from build123d import *

# Parameters (mm, degrees)
SKETCH_1_R          = 1.621125
EXTRUDE_403_DEPTH   = 3.2
SKETCH_2_OUTSIDE_W  = 36.28
SKETCH_2_OUTSIDE_H  = 37.362
SKETCH_2_OUTSIDE_R  = 3.5
CUT_EXTRUDE_1_DEPTH = 7.23083729
CUT_EXTRUDE_1_DRAFT = -60
SKETCH_3_OUTSIDE_W  = 36.28
SKETCH_3_OUTSIDE_H  = 37.362
SKETCH_3_OUTSIDE_R  = 3.5
CUT_EXTRUDE_2_DEPTH = 7.23083729
CUT_EXTRUDE_2_DRAFT = -60


with BuildPart() as part:
    # 草图1 → Extrude 403 (new body)
    with BuildSketch(Plane.XY):
        Polygon((0, 4.041451884), (-3.5, 2.020725942), (-3.5, -2.020725942), (0, -4.041451884), (3.5, -2.020725942), (3.5, 2.020725942), align=None)
        Circle(SKETCH_1_R, mode=Mode.SUBTRACT)
    extrude(amount=EXTRUDE_403_DEPTH)


with BuildPart() as cut_extrude_1_tool:
    # 草图2 outside → 切除-拉伸1 (with draft: the straight prism first)
    with BuildSketch(Plane(origin=(0, 0, 0), x_dir=(-1, 0, 0), z_dir=(0, 0, -1))):
        Rectangle(SKETCH_2_OUTSIDE_W, SKETCH_2_OUTSIDE_H)
        Circle(SKETCH_2_OUTSIDE_R, mode=Mode.SUBTRACT)
    extrude(amount=-CUT_EXTRUDE_1_DEPTH)
    # 切除-拉伸1: the draft: its side faces are tilted about the plane it starts from
    cut_extrude_1_sides = [cut_extrude_1_tool.faces().sort_by_distance(p)[0] for p in [
        (0, -18.681, 3.615418645),
        (-18.14, 0, 3.615418645),
        (0, 18.681, 3.615418645),
        (18.14, 0, 3.615418645),
        (3.5, 0, 3.615418645),
    ]]
    draft(cut_extrude_1_sides, Plane(origin=(0, 0, 0), x_dir=(-1, 0, 0), z_dir=(0, 0, -1)), CUT_EXTRUDE_1_DRAFT)


with BuildPart() as part_1:
    add(part.part)

    # 切除-拉伸1: cut by cut_extrude_1_tool
    add(cut_extrude_1_tool.part, mode=Mode.SUBTRACT)


with BuildPart() as cut_extrude_2_tool:
    # 草图3 outside → 切除-拉伸2 (with draft: the straight prism first)
    with BuildSketch(Plane.XY.offset(3.2)):
        Rectangle(SKETCH_3_OUTSIDE_W, SKETCH_3_OUTSIDE_H)
        Circle(SKETCH_3_OUTSIDE_R, mode=Mode.SUBTRACT)
    extrude(amount=-CUT_EXTRUDE_2_DEPTH)
    # 切除-拉伸2: the draft: its side faces are tilted about the plane it starts from
    cut_extrude_2_sides = [cut_extrude_2_tool.faces().sort_by_distance(p)[0] for p in [
        (0, -18.681, -0.415418645),
        (18.14, 0, -0.415418645),
        (0, 18.681, -0.415418645),
        (-18.14, 0, -0.415418645),
        (-3.5, 0, -0.415418645),
    ]]
    draft(cut_extrude_2_sides, Plane.XY.offset(3.2), CUT_EXTRUDE_2_DRAFT)


with BuildPart() as part_2:
    add(part_1.part)

    # 切除-拉伸2: cut by cut_extrude_2_tool
    add(cut_extrude_2_tool.part, mode=Mode.SUBTRACT)


solid = part_2.part
Here's how the part is built. I have some questions about the finished solid (model axes, mm). Round coordinates to 2 decimals unless told otherwise and drop trailing zeros. Loops run counter-clockwise (first coordinate to the right, second up) from the corner with the lowest first, then second, coordinate; pieces in that order, holes last. Notation, with made-up numbers: (28.25, -33) -> (33.25, -33) arc R24 ccw to (33.25, -20) -> close; hole circle Ø9 at (-20, 69.5). An arc over 180 degrees is marked (long way). Write each question's results on one line, items separated by ' | '.
(1) If we section it at A-A, the plane z = 0.5: List the corners of the cut face in (x, y) for me, then the cut area to 3 significant figures.
Worked answers:
outline: (-3.5, -2.02) -> (0, -4.04) -> (3.5, -2.02) -> (3.5, 2.02) -> (0, 4.04) -> (-3.5, 2.02) -> close; hole circle Ø3.24 at (0, 0) | area: 34.2 mm2
(2) For P1, Ø1.5, axis at x = -0.5, z = 0.5, coming from the -Y side, with a flat end and sliding along its axis, tell me the tip position at first contact or that it passes through.
Worked answers:
P1: y = -4.04
(3) We'd pull the mould along Z, two halves only. Please class faces 1 (the face through (1.8, 3, 1.6)), 2 (the face through (-3.19, 1.85, 3.09)), 3 (the face through (3.19, 1.85, 0.11)): released by +Z, released by -Z, zero draft, split by the parting line, or undercut.
Worked answers:
face 1: zero draft | face 2: released by +Z | face 3: released by -Z
(4) If I drill on L1, parallel to Y at x = 0.5, z = 2.55; L2, parallel to Y at x = -1, z = 2.4; L3, parallel to X at y = 1.25, z = 0.4, over which ranges is the centre line in solid material (lowest first)?
Worked answers:
L1: -3.75 to -1.54, 1.54 to 3.75 | L2: -3.46 to -1.28, 1.28 to 3.46 | L3: -3.5 to -1.03, 1.03 to 3.5
